For this review, take the finished solid that the model builds, in its own axes (mm). A direction names the side the tool comes from. Give positions to 0.01 mm unless a question says otherwise; leave off trailing zeros. Return JSON: item names as keys, results as strings. Group by question number.
1) For faces 4 (the face through (0, -6, -182)), 5 (the face through (6, 20, -182)), list the 3-axis set-ups (+Z, -Z, +X, -X, +Y, -Y) from which the entire face can be reached by the end or side of a thin tool; tool diameter is ignored.
2) Add section A-A (z = -274). State how many separate pieces and enclosed holes the cut face has, then the cut area to 3 significant figures.
3) Insertion check: P1, Ø5, axis at y = -10, z = -299, coming from the +X side; P2, Ø0.7, axis at x = -2, z = -112.5, coming from the -Y side; P3, Ø4.5, axis at x = -0.5, z = -141, coming from the +Y side. Each pin has a flat end and moves straight along its axis. Give the tip position at first contact, or say it passes through.
4) The part is to be moulded in two halves that separate along Y. For faces 1 (the face through (0, 6, -182)), 2 (the face through (6, -20, -182)), 3 (the face through (10, 16, -182)), say which applies: released by +Y, released by -Y, zero draft, split by the parting line, or undercut.
5) To check wall thickness, follow line 1 along Y through (x, z) = (0, -91.5); line 2 along X through (y, z) = (5, -96.5); line 3 along X through (y, z) = (10, -285). State the ranges of each line that lie inside material, in increasing order.
Autodesk Inventor part; units mm, degrees
ref_plane "C1_XY" through (0, 0, 0) normal (0, 0, 1) x (1, 0, 0)
ref_plane "C1_YZ" through (0, 0, 0) normal (1, 0, 0) x (0, 1, 0)
ref_plane "C1_ZX" through (0, 0, 0) normal (0, 1, 0) x (0, 0, 1)
sketch "Sketch_1" plane through (0, 0, 0) normal (0, 0, 1) x (1, 0, 0)
  line L0 (-10, -7) -> (-8, -7)
  line L1 (-8, -7) -> (-8, -4)
  line L2 (-8, -4) -> (-7.0607, -4)
  line L3 (-7.0607, -4) -> (-4, -7.0607)
  line L4 (-4, -7.0607) -> (-4, -9.4804)
  line L5 (-4, -9.4804) -> (-3.7, -10)
  line L6 (-3.7, -10) -> (-4, -10.5196)
  line L7 (-4, -10.5196) -> (-4, -12.9393)
  line L8 (-4, -12.9393) -> (-7.0607, -16)
  line L9 (-7.0607, -16) -> (-8, -16)
  line L10 (-8, -16) -> (-8, -13)
  line L11 (-8, -13) -> (-10, -13)
  line L12 (-10, -13) -> (-10, -19)
  arc A0 (-10, -19) -> (-9, -20) centre (-9, -19) ccw
  line L13 (-9, -20) -> (-3, -20)
  line L14 (-3, -20) -> (-3, -18)
  line L15 (-3, -18) -> (-6, -18)
  line L16 (-6, -18) -> (-6, -17.0607)
  line L17 (-6, -17.0607) -> (-2.9393, -14)
  line L18 (-2.9393, -14) -> (-0.5196, -14)
  line L19 (-0.5196, -14) -> (0, -13.7)
  line L20 (0, -13.7) -> (0.5196, -14)
  line L21 (0.5196, -14) -> (2.9393, -14)
  line L22 (2.9393, -14) -> (6, -17.0607)
  line L23 (6, -17.0607) -> (6, -18)
  line L24 (6, -18) -> (3, -18)
  line L25 (3, -18) -> (3, -20)
  line L26 (3, -20) -> (9, -20)
  arc A1 (9, -20) -> (10, -19) centre (9, -19) ccw
  line L27 (10, -19) -> (10, -13)
  line L28 (10, -13) -> (8, -13)
  line L29 (8, -13) -> (8, -16)
  line L30 (8, -16) -> (7.0607, -16)
  line L31 (7.0607, -16) -> (4, -12.9393)
  line L32 (4, -12.9393) -> (4, -10.5196)
  line L33 (4, -10.5196) -> (3.7, -10)
  line L34 (3.7, -10) -> (4, -9.4804)
  line L35 (4, -9.4804) -> (4, -7.0607)
  line L36 (4, -7.0607) -> (7.0607, -4)
  line L37 (7.0607, -4) -> (8, -4)
  line L38 (8, -4) -> (8, -7)
  line L39 (8, -7) -> (10, -7)
  line L40 (10, -7) -> (10, 7)
  line L41 (10, 7) -> (8, 7)
  line L42 (8, 7) -> (8, 4)
  line L43 (8, 4) -> (7.0607, 4)
  line L44 (7.0607, 4) -> (4, 7.0607)
  line L45 (4, 7.0607) -> (4, 9.4804)
  line L46 (4, 9.4804) -> (3.7, 10)
  line L47 (3.7, 10) -> (4, 10.5196)
  line L48 (4, 10.5196) -> (4, 12.9393)
  line L49 (4, 12.9393) -> (7.0607, 16)
  line L50 (7.0607, 16) -> (8, 16)
  line L51 (8, 16) -> (8, 13)
  line L52 (8, 13) -> (10, 13)
  line L53 (10, 13) -> (10, 19)
  arc A2 (10, 19) -> (9, 20) centre (9, 19) ccw
  line L54 (9, 20) -> (3, 20)
  line L55 (3, 20) -> (3, 18)
  line L56 (3, 18) -> (6, 18)
  line L57 (6, 18) -> (6, 17.0607)
  line L58 (6, 17.0607) -> (2.9393, 14)
  line L59 (2.9393, 14) -> (0.5196, 14)
  line L60 (0.5196, 14) -> (0, 13.7)
  line L61 (0, 13.7) -> (-0.5196, 14)
  line L62 (-0.5196, 14) -> (-2.9393, 14)
  line L63 (-2.9393, 14) -> (-6, 17.0607)
  line L64 (-6, 17.0607) -> (-6, 18)
  line L65 (-6, 18) -> (-3, 18)
  line L66 (-3, 18) -> (-3, 20)
  line L67 (-3, 20) -> (-9, 20)
  arc A3 (-9, 20) -> (-10, 19) centre (-9, 19) ccw
  line L68 (-10, 19) -> (-10, 13)
  line L69 (-10, 13) -> (-8, 13)
  line L70 (-8, 13) -> (-8, 16)
  line L71 (-8, 16) -> (-7.0607, 16)
  line L72 (-7.0607, 16) -> (-4, 12.9393)
  line L73 (-4, 12.9393) -> (-4, 10.5196)
  line L74 (-4, 10.5196) -> (-3.7, 10)
  line L75 (-3.7, 10) -> (-4, 9.4804)
  line L76 (-4, 9.4804) -> (-4, 7.0607)
  line L77 (-4, 7.0607) -> (-7.0607, 4)
  line L78 (-7.0607, 4) -> (-8, 4)
  line L79 (-8, 4) -> (-8, 7)
  line L80 (-8, 7) -> (-10, 7)
  line L81 (-10, 7) -> (-10, -7)
  line L82 (-8, 1.7) -> (-8, -1.7)
  arc A4 (-8, -1.7) -> (-7.7, -2) centre (-7.7, -1.7) ccw
  line L83 (-7.7, -2) -> (-7.0636, -2)
  arc A5 (-6.8515, -2.0879) -> (-7.0636, -2) centre (-7.0636, -2.3) ccw
  line L84 (-6.8515, -2.0879) -> (-2.9393, -6)
  line L85 (-2.9393, -6) -> (2.9393, -6)
  line L86 (2.9393, -6) -> (6.8515, -2.0879)
  arc A6 (7.0636, -2) -> (6.8515, -2.0879) centre (7.0636, -2.3) ccw
  line L87 (7.0636, -2) -> (7.7, -2)
  arc A7 (7.7, -2) -> (8, -1.7) centre (7.7, -1.7) ccw
  line L88 (8, -1.7) -> (8, 1.7)
  arc A8 (8, 1.7) -> (7.7, 2) centre (7.7, 1.7) ccw
  line L89 (7.7, 2) -> (7.0636, 2)
  arc A9 (6.8515, 2.0879) -> (7.0636, 2) centre (7.0636, 2.3) ccw
  line L90 (6.8515, 2.0879) -> (2.9393, 6)
  line L91 (2.9393, 6) -> (-2.9393, 6)
  line L92 (-2.9393, 6) -> (-6.8515, 2.0879)
  arc A10 (-7.0636, 2) -> (-6.8515, 2.0879) centre (-7.0636, 2.3) ccw
  line L93 (-7.0636, 2) -> (-7.7, 2)
  arc A11 (-7.7, 2) -> (-8, 1.7) centre (-7.7, 1.7) ccw
extrude "Extrusion1" add sketch "Sketch_1" against normal blind 370
sketch "Sketch2" plane through (0, 0, -370) normal (0, 0, -1) x (-1, 0, 0)
  point P0 (0, 10)
hole "Hole1" at (0, 10, -370) direction (0, 0, 1) diameter 4.2 depth 370
pattern_linear "Rectangular Pattern1" count 2 spacing 20 along (0, -1, 0) of "Hole1"
ref_plane "C1_XY" through (0, 0, 0) normal (0, 0, 1) x (1, 0, 0)
ref_plane "C1_YZ" through (0, 0, 0) normal (1, 0, 0) x (0, 1, 0)
ref_plane "C1_ZX" through (0, 0, 0) normal (0, 1, 0) x (0, 0, 1)
properties part number "HFS5-2040-370"
Evaluation:
{
 "1": {"face 4": "+Z, -Z", "face 5": "+Z, -Z, +X, -X, +Y"},
 "2": {"separate pieces": "1", "enclosed holes": "3", "area": "324 mm^2"},
 "3": {"P1": "x = 4", "P2": "y = -14", "P3": "y = 14"},
 "4": {"face 1": "undercut", "face 2": "released by -Y", "face 3": "zero draft"},
 "5": {"line 1": "-13.7 to -12.1, -7.9 to -6, 6 to 7.9, 12.1 to 13.7", "line 2": "-10 to -8, -6.06 to -3.94, 3.94 to 6.06, 8 to 10", "line 3": "-3.7 to -2.1, 2.1 to 3.7"}
}
